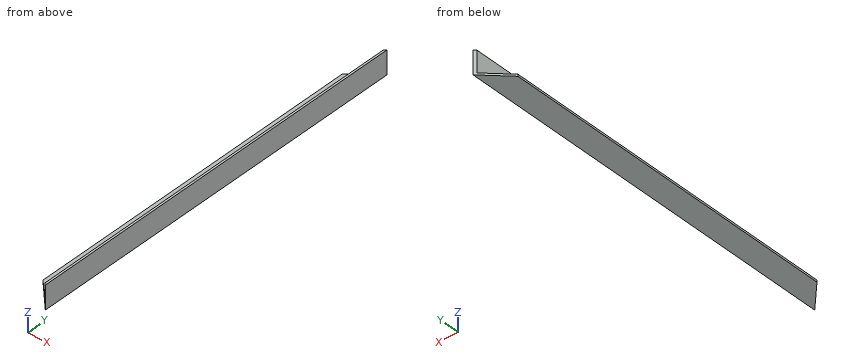
```python
from build123d import *

# Parameters (mm, degrees)
F1_DEPTH = 1219.2
F3_DEPTH = 76.2


with BuildPart() as f1:
    # F0 (on Front) → F1 (new body)
    with BuildSketch(Plane.XZ):
        Polygon((0, 0), (0, 76.2), (-6.35, 76.2), (-6.35, 6.35), (-76.2, 6.35), (-76.2, 0), align=None)
    extrude(amount=-F1_DEPTH)

    # F2 (on face) → F3 (cut)
    with BuildSketch(Plane.XY.offset(76.2)):
        Polygon((0, 1219.2), (-76.2, 1219.2), (-76.2, 1143), align=None)
        Polygon((-76.2, 0), (0, 0), (-76.2, 76.2), align=None)
    extrude(amount=-F3_DEPTH, mode=Mode.SUBTRACT)


solid = f1.part
```
CAD build for the part. Positions are in the model's coordinates, mm. Coordinates: 2 decimals unless noted, no trailing zeros. Loops run counter-clockwise (first coordinate to the right, second up) from the corner with the lowest first, then second, coordinate; pieces in that order, holes last. Notation, with made-up numbers: (-9, 81.5) - (11, 81.5) arc R9 cw to (11, 98.5) - close; hole circle Ø9 at (18.25, -22). An arc over 180 degrees is marked (long way). Use CSV: the item, a comma, the result in double quotes. Start each with the question number.
Q1. Drop flat-ended pins along their axis: P1, Ø10, axis at x = -67.5, y = 889, coming from the +Z side; P2, Ø5, axis at y = 620.5, z = 16.5, coming from the -X side. Give the stop position or say it passes through.
Q2. Probe probe 1 along Z at (x, y) = (-46, 79); probe 2 along X at (y, z) = (610.5, 55). List the from-to ranges inside material, lowest first. Write a range as from..to.
Q3. Cut at A-A, the plane y = 569.5. List the corners of the cut face in (x, z).
Q4. Cut at B-B, the plane x = -45.5. List the corners of the cut face in (y, z), then the cut area to 3 significant figures.
Q5. Cut at C-C, the plane z = 47.5. List the corners of the cut face in (x, y), then the cut area to 3 significant figures.
Here are the results:
1,P1,"z = 6.35"
1,P2,"x = -6.35"
2,probe 1,"0..6.35"
2,probe 2,"-6.35..0"
3,outline,"(-76.2, 0) - (0, 0) - (0, 76.2) - (-6.35, 76.2) - (-6.35, 6.35) - (-76.2, 6.35) - close"
4,outline,"(45.5, 0) - (1173.7, 0) - (1173.7, 6.35) - (45.5, 6.35) - close"
4,area,"7,160 mm2"
5,outline,"(-6.35, 6.35) - (0, 0) - (0, 1219.2) - (-6.35, 1212.85) - close"
5,area,"7,700 mm2"
